Could you check a few things on this model? Use its own coordinates, in mm. Face numbers are marked on the shaded views. A direction names the side the tool comes from. Round coordinates to 2 decimals unless told otherwise and drop trailing zeros. Write each loop counter-clockwise with the first axis right and the second up, starting at its lowest first coordinate (ties: lowest second). Pieces come first, ordered by that corner, then holes. Notation, with made-up numbers: (52.5, -36) - (82.5, -36) arc R24 ccw to (82.5, -15) - close; hole circle Ø7 at (-38, 12). An arc over 180 degrees is marked (long way). Put each result on its own line as item: value.
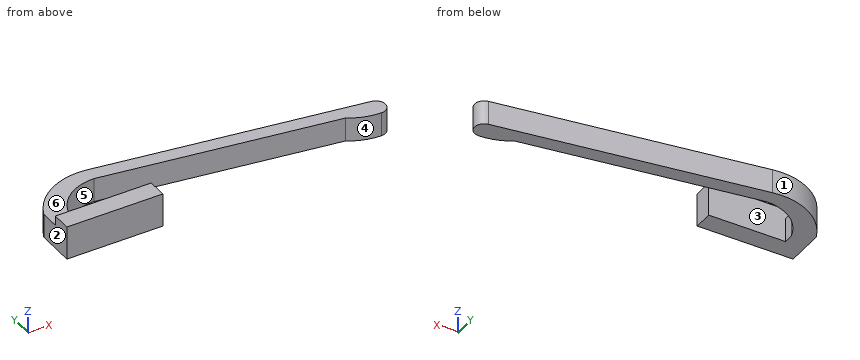
from build123d import *

# Parameters (mm, degrees)
F1_DEPTH = 5
F2_DEPTH = 7


with BuildPart() as f1:
    # F0 (on Top) → F1 (new body)
    with BuildSketch(Plane.XY):
        with BuildLine():
            ThreePointArc((61.629022, 5.913021), (64.679214, 4.488544), (68.009999, 4))
            ThreePointArc((68.009999, 4), (70.004837, 5.856404), (68.29645, 7.97938))
            Line((68.29645, 7.97938), (13.861023, 15.857132))
            ThreePointArc((13.861023, 15.857132), (5.586179, 14.300147), (0, 8))
            Line((0, 8), (0, 4))
            Line((0, 4), (4, 4))
            Line((4, 4), (4, 6))
            ThreePointArc((4, 6), (7.547234, 11.043894), (13.431347, 12.888062))
            Line((13.431347, 12.888062), (61.629022, 5.913021))
        make_face()
    extrude(amount=F1_DEPTH)

    # F0 (on Top) → F2 (join)
    with BuildSketch(Plane.XY):
        Polygon((4, 4), (0, 4), (0, 0), (20, 0), (20, 4), align=None)
    extrude(amount=F2_DEPTH)


solid = f1.part
(1) If we mould it in two halves opening along Y, with no side actions, what happens to the marked faces 1, 2 and 3? For each: pulls with the +Y half, pulls with the -Y half, needs draft (parallel to the pull), parting line crosses it, or undercut.
Values found:
face 1: pulls with the +Y half
face 2: needs draft
face 3: undercut
(2) For the marked faces 4, 5 and 6, which set-ups out of +Z, -Z, +X, -X, +Y, -Y let a thin tool reach every point of the face, with its end or its side?
Values found:
face 4: +Z, -Z, -Y
face 5: +Z, -Z
face 6: +Z, +X, -X, +Y
(3) Imagine slicing it at C-C, the plane x = 5. List the corners of the cut face in (y, z) for me.
Values found:
outline: (0, 0) - (4, 0) - (4, 7) - (0, 7) - close; (8.27, 0) - (13.95, 0) - (13.95, 5) - (8.27, 5) - close
(4) Imagine slicing it at B-B, the plane z = 1. List the corners of the cut face in (x, y) for me, then the cut area to 3 significant figures.
Values found:
outline: (0, 0) - (20, 0) - (20, 4) - (4, 4) - (4, 6) arc R9.6 cw to (13.43, 12.89) - (61.63, 5.91) arc R11.6 ccw to (68.01, 4) arc R2 ccw to (68.3, 7.98) - (13.86, 15.86) arc R13 ccw to (0, 8) - close
area: 324 mm^2
(5) Imagine slicing it at D-D, the plane y = 1.75. List the corners of the cut face in (x, z) for me.
Values found:
outline: (0, 0) - (20, 0) - (20, 7) - (0, 7) - close
(6) I'm going to push flat-ended pins straight in: pin 1 (1.6 mm diameter, centred on y = 5, z = 2.5, fed in from +X); pin 2 (1.5 mm diameter, centred on y = 9.5, z = 3, fed in from -X); pin 3 (2 mm diameter, centred on x = 13.5, z = 3.5, fed in from +Y). Where does each tip first touch, or does it pass through?
Values found:
pin 1: stops at x = 70
pin 2: stops at x = 0.34
pin 3: stops at y = 15.98
(7) Imagine slicing it at A-A, the plane y = 7.25. List the corners of the cut face in (x, z) for me.
Values found:
outline: (0, 0) - (4.46, 0) - (4.46, 5) - (0, 5) - close; (52.39, 0) - (69.57, 0) - (69.57, 5) - (52.39, 5) - close
(8) Please list where these lines run through material, in increasing order: probe 1 along Z at (x, y) = (53.5, 7.25); probe 2 along X at (y, z) = (3.5, 4); probe 3 along Y at (x, z) = (7.5, 5.75). Write a range as from..to.
Values found:
probe 1: z = 0..5
probe 2: x = 0..20
probe 3: y = 0..4
